Here's the drawing with two shaded views (mm, measured from the low corner). I have some questions. A direction names the side the tool comes from. Give positions to 0.01 mm unless a question says otherwise; leave off trailing zeros. Order: outer loops, then holes, each group sorted by start corner. A loop starts at its lowest first (then second) coordinate and runs counter-clockwise, first axis right, second up. Notation, with made-up numbers: (81, 50.5) - (94, 50.5) arc R22 ccw to (94, 78.5) - close; hole circle Ø8 at (40.25, -5). An arc over 180 degrees is marked (long way). Use one line per item in the form item = value. Start each with the question number.
1) Suppose I cut it at C-C, the plane x = 5.25. Write out the boundary of the cut face in (y, z) (1 decimal).
2) For pin 1 (1.1 mm diameter, centred on x = 0.5, z = 7, fed in from +Y); pin 2 (1 mm diameter, centred on y = 13.5, z = 6, fed in from -X); pin 3 (1.1 mm diameter, centred on y = 24.5, z = 18.5, fed in from -X), each with a flat end and sliding along its axis, tell me the tip position at first contact or that it passes through.
3) Please list where these lines run through material, in increasing order: probe 1 along Y at (x, z) = (12.7, 5.5); probe 2 along X at (y, z) = (8.25, 5) (1 decimal); probe 3 along Y at (x, z) = (6.5, 11.5) (1 decimal).
4) Suppose I cut it at A-A, the plane x = 12.7. Write out the boundary of the cut face in (y, z).
5) Suppose I cut it at D-D, the plane y = 4.25. Write out the boundary of the cut face in (x, z) (1 decimal), and give its area (3 significant figures).
6) We'd pull the mould along X, two halves only. Please class the marked faces 1, 2 and 3: released by +X, released by -X, zero draft, split by the parting line, or undercut.
7) Which directions (+Z, -Z, +X, -X, +Y, -Y) give clear straight access to the entire face, cutting with the end or side of a thin tool? Please do the marked faces 4, 5, 6, 7 and 8.
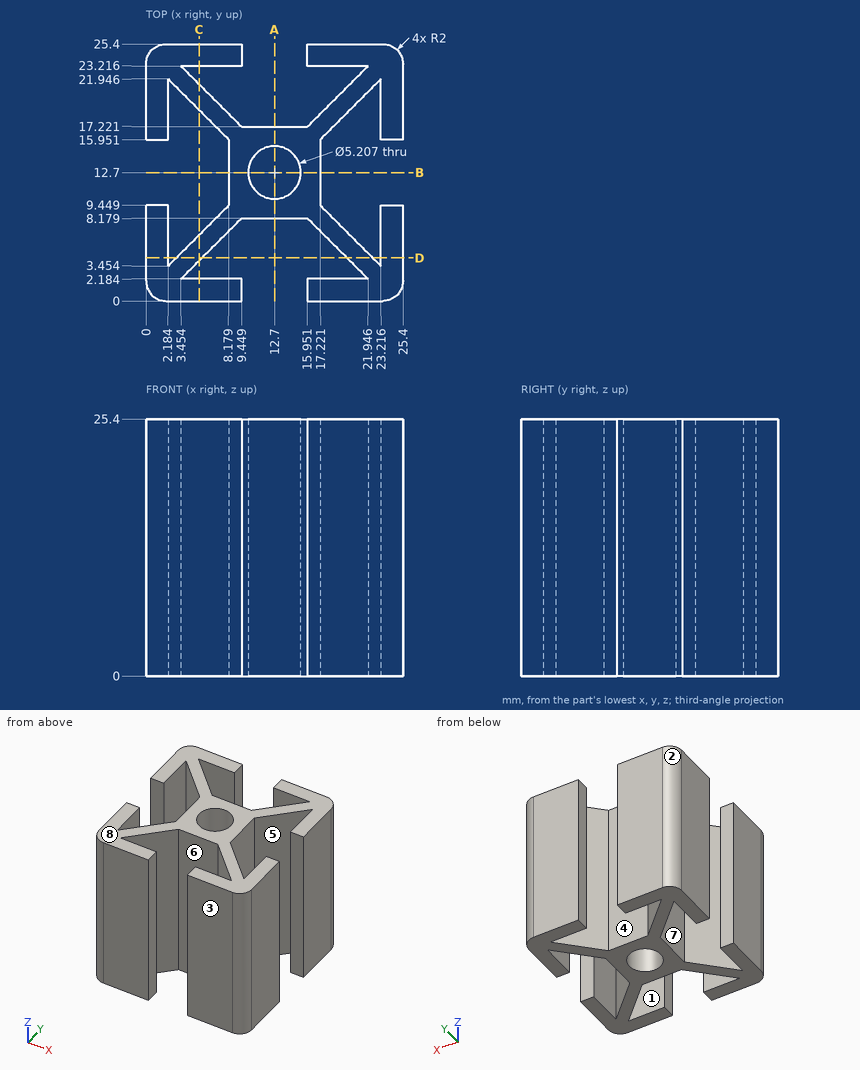
Result sheet:
q1.outline = (0, 0) - (2.2, 0) - (2.2, 25.4) - (0, 25.4) - close; (4, 0) - (6.5, 0) - (6.5, 25.4) - (4, 25.4) - close; (18.9, 0) - (21.4, 0) - (21.4, 25.4) - (18.9, 25.4) - close; (23.2, 0) - (25.4, 0) - (25.4, 25.4) - (23.2, 25.4) - close
q2.pin_1 = 25.16
q2.pin_2 = 8.18
q2.pin_3 = 0.08
q3.probe_1 = 8.18 to 10.1, 15.3 to 17.22
q3.probe_2 = 0 to 2.2, 7 to 18.4, 23.2 to 25.4
q3.probe_3 = 0 to 2.2, 5.2 to 7.8, 17.6 to 20.2, 23.2 to 25.4
q4.outline = (8.18, 0) - (10.1, 0) - (10.1, 25.4) - (8.18, 25.4) - close; (15.3, 0) - (17.22, 0) - (17.22, 25.4) - (15.3, 25.4) - close
q5.outline = (0, 0) - (2.2, 0) - (2.2, 25.4) - (0, 25.4) - close; (3, 0) - (5.5, 0) - (5.5, 25.4) - (3, 25.4) - close; (19.9, 0) - (22.4, 0) - (22.4, 25.4) - (19.9, 25.4) - close; (23.2, 0) - (25.4, 0) - (25.4, 25.4) - (23.2, 25.4) - close
q5.area = 240 mm²
q6.face_1 = undercut
q6.face_2 = released by -X
q6.face_3 = zero draft
q7.face_4 = +Z, -Z, +Y
q7.face_5 = +Z, -Z
q7.face_6 = +Z, -Z, -Y
q7.face_7 = +Z, -Z, -X
q7.face_8 = +Z, +X, -X, +Y, -Y
